Verification items for the finished model (mm, model axes). Coordinates: 2 decimals unless noted, no trailing zeros. Write each loop counter-clockwise with the first axis right and the second up, starting at its lowest first coordinate (ties: lowest second). Pieces come first, ordered by that corner, then holes. Notation, with made-up numbers: (20.5, -19) -> (51.5, -19) arc R19 cw to (51.5, 14) -> close; hole circle Ø6 at (69, -11). An arc over 180 degrees is marked (long way). Answer in a Markdown table with one row per item.
```python
from build123d import *

# Parameters (mm, degrees)
BOSS_EXTRUDE1_DEPTH = 25
FILLET1_R           = 12.5
CUT_EXTRUDE1_REACH  = 175.866
SKETCH3_R           = 7.89
SKETCH4_R           = 3.225
BOSS_EXTRUDE2_DEPTH = 6


with BuildPart() as part:
    # Sketch2 → Boss-Extrude1 (new body)
    with BuildSketch(Plane.XY):
        with BuildLine():
            Line((0, 108), (-25, 108))
            Line((-25, 108), (-25, 105))
            Line((-25, 105), (0, 105))
            ThreePointArc((0, 105), (74.56946444, 73.921546068), (104.996001922, -0.916286227))
            Line((104.996001922, -0.916286227), (104.777838534, -25.915334304))
            Line((104.777838534, -25.915334304), (107.777724303, -25.94151391))
            Line((107.777724303, -25.94151391), (107.995887691, -0.942465834))
            ThreePointArc((107.995887691, -0.942465834), (76.700020567, 76.033590241), (0, 108))
        make_face()
    extrude(amount=BOSS_EXTRUDE1_DEPTH)

    # Fillet1
    fillet1_edges = [part.edges().sort_by_distance(p)[0] for p in [
        (106.277781419, -25.928424107, 0),
        (106.277781419, -25.928424107, 25),
        (-25, 106.5, 25),
        (-25, 106.5, 0),
    ]]
    fillet(fillet1_edges, radius=FILLET1_R - 0.0001)  # a hair under: the kernel refuses the full size

    # Sketch3 → Cut-Extrude1 (cut, up to next)
    with BuildSketch(Plane(origin=(0, 108, 0), x_dir=(1, 0, 0), z_dir=(0, 1, 0)), mode=Mode.PRIVATE) as cut_extrude1_sk1:
        with Locations(Location((-12.5, -12.5, 0), (0, 0, 270))):
            Circle(SKETCH3_R)
    cut_extrude1_tool1 = extrude(cut_extrude1_sk1.sketch, amount=-CUT_EXTRUDE1_REACH, mode=Mode.PRIVATE) & part.part
    add(cut_extrude1_tool1.solids().sort_by_distance((-12.5, 108, 12.5))[0], mode=Mode.SUBTRACT)

    # Sketch4 → Boss-Extrude2 (add)
    with BuildSketch(Plane(origin=(104.996001922, -0.916286227, 0), x_dir=(0, 0, -1), z_dir=(0.9999619230641714, -0.008726535498378436, 0))):
        with Locations(Location((-12.5, -12.5, 0), (0, 0, 90))):
            Circle(SKETCH4_R)
    extrude(amount=-BOSS_EXTRUDE2_DEPTH)


solid = part.part
```
1. Go/stop test with flat-tipped pins: pin 1 (14 mm diameter, centred on x = -12.5, z = 12.5, fed in from -Y); pin 2 (3 mm diameter, centred on y = 78, z = 15.5, fed in from +X); pin 3 (3 mm diameter, centred on y = 85.5, z = 9.5, fed in from -X); pin 4 (1 mm diameter, centred on x = 61.5, z = 20.5, fed in from +Y). Record where each tip stops, or that it passes through.
Findings below:
| item | result |
|---|---|
| pin 1 | passes through |
| pin 2 | stops at x = 76.23 |
| pin 3 | stops at x = 58.79 |
| pin 4 | stops at y = 89.12 |
2. Sectioned sample at A-A, the plane y = 54. Record the cut outline in (x, z), and give its area (3 significant figures).
Findings below:
| item | result |
|---|---|
| outline | (90.05, 0) -> (93.53, 0) -> (93.53, 25) -> (90.05, 25) -> close |
| area | 87.0 mm² |
3. Release check for a two-part mould opening along Z. For faces 1 (the face through (-4, 105, 12)), 2 (the face through (-17.3, 106.52, 6.24)), 3 (the face through (79, 70, 0)), 4 (the face through (79, 70, 25)) record: released by +Z, released by -Z, zero draft, split by the parting line, or undercut.
Findings below:
| item | result |
|---|---|
| face 1 | zero draft |
| face 2 | undercut |
| face 3 | released by -Z |
| face 4 | released by +Z |
4. Material ranges on probe 1 along Z at (x, y) = (-12, 106); probe 2 along X at (y, z) = (7, 18.75); probe 3 along X at (y, z) = (-1, 15.25), recorded low to high. Write a range as from..to.
Findings below:
| item | result |
|---|---|
| probe 1 | z = 0..4.63, 20.37..25 |
| probe 2 | x = 104.77..107.77 |
| probe 3 | x = 105..108 |
